```python
from build123d import *

# Parameters (mm, degrees)
SKICA1_R                = 5
P_IDAT_VYSUNUT_M1_DEPTH = 8
ZAOBLIT1_R              = 30
ZAOBLIT2_R              = 1


with BuildPart() as part:
    # Skica1 → Přidat vysunutím1 (new body)
    with BuildSketch(Plane(origin=(0, 0, 0), x_dir=(0, 0, -1), z_dir=(1, 0, 0))):
        Polygon((-30, 110), (30, 110), (40, 0), (-40, 0), align=None)
        with Locations((0, 85)):
            Circle(SKICA1_R, mode=Mode.SUBTRACT)
        with Locations((0, 50)):
            Circle(SKICA1_R, mode=Mode.SUBTRACT)
    extrude(amount=P_IDAT_VYSUNUT_M1_DEPTH)

    # Zaoblit1
    zaoblit1_edges = [part.edges().sort_by_distance(p)[0] for p in [
        (4, 110, 30),
        (4, 110, -30),
    ]]
    fillet(zaoblit1_edges, radius=ZAOBLIT1_R)

    # Zaoblit2
    zaoblit2_edges = [part.edges().sort_by_distance(p)[0] for p in [
        (0, 110, 0),
        (8, 110, 0),
        (0, 41.358036191, 36.240178528),
        (0, 102.152676717, 22.833709509),
        (0, 102.152676717, -22.833709509),
        (8, 41.358036191, 36.240178528),
        (8, 102.152676717, 22.833709509),
        (8, 102.152676717, -22.833709509),
        (8, 41.358036191, -36.240178528),
        (0, 41.358036191, -36.240178528),
    ]]
    fillet(zaoblit2_edges, radius=ZAOBLIT2_R)


solid = part.part
```
Could you check a few things on this model? Use its own coordinates, in mm. Round coordinates to 2 decimals unless told otherwise and drop trailing zeros. Loops run counter-clockwise (first coordinate to the right, second up) from the corner with the lowest first, then second, coordinate; pieces in that order, holes last. Notation, with made-up numbers: M -34.75,11 L -13.75,11 A14 cw -13.75,30 Z; hole C 50.5,-19 d4. An arc over 180 degrees is marked long. Put each result on its own line as item: value.
Q1. Thinking about a two-plate mould opening in Z: for faces 1 (the face through (4, 102, -23)), 2 (the face through (0.301, 41.911, 35.904)), 3 (the face through (3.944, 54.957, 0.651)), 4 (the face through (3.94, 80.12, 1.08)), which applies, released by +Z, released by -Z, zero draft, split by the parting line, or undercut?
Check result:
face 1: released by -Z
face 2: released by +Z
face 3: undercut
face 4: undercut
Q2. Imagine slicing it at B-B (x = 3.75). Write out the boundary of the cut face in (y, z), then the cut area to 3 significant figures.
Check result:
outline: M 0,-40 L 82.72,-32.48 A30 ccw 110,-2.6 L 110,2.6 A30 ccw 82.72,32.48 L 0,40 Z; hole C 50,0 d10; hole C 85,0 d10
area: 7,230 mm2
Q3. Imagine slicing it at A-A (z = 0). Write out the boundary of the cut face in (x, y), then the cut area to 3 significant figures.
Check result:
outline: M 0,0 L 8,0 L 8,45 L 0,45 Z; M 0,55 L 8,55 L 8,80 L 0,80 Z; M 0,90 L 8,90 L 8,109 A1 ccw 7,110 L 1,110 A1 ccw 0,109 Z
area: 720 mm2
Q4. For pin 1 (2 mm diameter, centred on x = 3, z = -24, fed in from +Y), with a flat end and sliding along its axis, tell me the tip position at first contact or that it passes through.
Check result:
pin 1: y = 102
Q5. I need wall thicknesses on probe 1 along Y at (x, z) = (2.5, 0); probe 2 along Y at (x, z) = (2.5, 1); probe 3 along Y at (x, z) = (2, -21). Which ranges of each line are inside material? Lowest first, please.
Check result:
probe 1: 0 to 45, 55 to 80, 90 to 110
probe 2: 0 to 45.1, 54.9 to 80.1, 89.9 to 110
probe 3: 0 to 103.7
